Geometry check sheet. Reference: the model listing, model coordinates, mm. A direction names the side the tool comes from. Coordinates: 2 decimals unless noted, no trailing zeros. Loops run counter-clockwise (first coordinate to the right, second up) from the corner with the lowest first, then second, coordinate; pieces in that order, holes last. Notation, with made-up numbers: M -25.75,-26 L 3.25,-26 A7 cw 3.25,-21 Z; hole C 29,-3 d7. An arc over 180 degrees is marked long. Use CSV: the item, a comma, the result in double quotes.
```python
from build123d import *

# Parameters (mm, degrees)
BOSS_EXTRUDE1_DEPTH = 49


with BuildPart() as part:
    # Sketch1 → Boss-Extrude1 (new body, symmetric)
    with BuildSketch(Plane(origin=(0, 0, 0), x_dir=(0, 0, -1), z_dir=(1, 0, 0))):
        Polygon((-61.102982905, 46.194785918), (-62.332373369, 50.782933593), (-64.264225021, 50.265295502), (-49.991832107, -3), (-35, -17), (8, -17), (8, 7.5), (-3, 7.5), (-14, 0), (-32.467253687, 0), (-57.53744343, 47.150169341), align=None)
    extrude(amount=BOSS_EXTRUDE1_DEPTH, both=True)


solid = part.part
```
1. Release check for a two-part mould opening along Z. For faces 4 (the flat face through (1, -5, -8)), 5 (the flat face through (1, 0, 23)), 6 (the flat face through (0.69, 24.01, 57.23)), 7 (the flat face through (49, -1, 31)) record: +Z half, -Z half, draft (parallel to the pull), parting line (faces both ways), or undercut.
The answers:
face 4,"-Z half"
face 5,"undercut"
face 6,"+Z half"
face 7,"draft"
2. Gauge pin test, flat ends, axial feed: P1, Ø5, axis at x = -19.5, z = 51.5, coming from the +Y side; P2, Ø9, axis at x = 23.5, z = 22.5, coming from the +Y side; P3, Ø3.5, axis at x = 3.5, z = -1, coming from the +Y side. Record the tip position at first contact, or that the pin passes through.
The answers:
P1,"y = 40.5"
P2,"y = 0"
P3,"y = 7.5"
3. Section check A-A, the plane x = 8.5. Record the cut outline in (y, z).
The answers:
outline,"M -17,-8 L 7.5,-8 L 7.5,3 L 0,14 L 0,32.47 L 47.15,57.54 L 46.19,61.1 L 50.78,62.33 L 50.27,64.26 L -3,49.99 L -17,35 Z"
4. Section check C-C, the plane z = 30.5. Record the cut outline in (x, y).
The answers:
outline,"M -49,-17 L 49,-17 L 49,0 L -49,0 Z"
5. Thickness scan on line 1 (Z direction, x = 7.5, y = -2); line 2 (Y direction, x = -11, z = -1); line 3 (Z direction, x = -8.5, y = 14). Record the ranges inside material, lowest first. Write a range as [from, to].
The answers:
line 1,"[-8, 50.26]"
line 2,"[-17, 7.5]"
line 3,"[39.91, 54.55]"
6. Section check B-B, the plane y = 3. Record the cut outline in (x, z).
The answers:
outline,"M -49,-8 L 49,-8 L 49,9.6 L -49,9.6 Z; M -49,34.06 L 49,34.06 L 49,51.6 L -49,51.6 Z"
7. Section check D-D, the plane y = 12. Record the cut outline in (x, z).
The answers:
outline,"M -49,38.85 L 49,38.85 L 49,54.01 L -49,54.01 Z"
8. Set-up check for faces 1 (the flat face through (0.69, 48.46, 61.71)), 2 (the flat face through (0.686, -9.902, 42.601)), 3 (the flat face through (1, 7.5, -3)): record each of +Z, -Z, +X, -X, +Y, -Y from which the full face is reachable in a straight line by a thin tool's end or side.
The answers:
face 1,"+X, -X, +Y"
face 2,"+Z, +X, -X, -Y"
face 3,"-Z, +X, -X, +Y"
